```python
from build123d import *

# Parameters (mm, degrees)
SKETCH_1_W      = 160
SKETCH_1_H      = 100
EXTRUDE_4_DEPTH = 20
SKETCH_3_R      = 20
EXTRUDE_5_DEPTH = 35


with BuildPart() as part:
    # 草图1 → 凸台-拉伸4 (new body)
    with BuildSketch(Plane.XY):
        with Locations((-86.209434593, 50.003007896)):
            Rectangle(SKETCH_1_W, SKETCH_1_H)
    extrude(amount=-EXTRUDE_4_DEPTH)

    # 草图3 → 凸台-拉伸5 (add)
    with BuildSketch(Plane(origin=(0, 0, -20), x_dir=(-1, 0, 0), z_dir=(0, 0, -1))):
        with Locations(Location((46.209434593, 50.003007896, 0), (0, 0, 180))):
            Circle(SKETCH_3_R)
        with Locations(Location((126.209434593, 50.003007896, 0), (0, 0, 180))):
            Circle(SKETCH_3_R)
    extrude(amount=EXTRUDE_5_DEPTH)


solid = part.part
```
Source: CAD feature listing. Evaluate the final solid. Frame: model axes, mm. A direction names the side the tool comes from. Round coordinates to 2 decimals unless told otherwise and drop trailing zeros. Loops run counter-clockwise (first coordinate to the right, second up) from the corner with the lowest first, then second, coordinate; pieces in that order, holes last. Notation, with made-up numbers: M -34.75,80.5 L -25.75,80.5 A19 cw -25.75,111.5 Z; hole C -2,68 d4. An arc over 180 degrees is marked long. Use a Markdown table: item, result. Add a question column.
1. Cut plane D-D, the plane y = 32. Output: boundary loops of the cut face in (x, z).
2. Ray query, line 1 along Z through (x, y) = (-89.5, 66); line 2 along X through (y, z) = (52, -31); line 3 along X through (y, z) = (59, -25). Return the intervals inside material, ascending. Write a range as [from, to].
3. Cut plane B-B, the plane x = -120. Output: boundary loops of the cut face in (y, z).
4. Pull-direction query (X, two-part tool) for faces 3 (the flat face through (-87, 100.003, -10)), 4 (the flat face through (-166.209, 49, -10)), 5 (the cylindrical face through (-146.19, 49.12, -37.25)); classes: +X half, -X half, draft (parallel to the pull), parting line (faces both ways), or undercut.
5. Contact query for flat-ended pins moving along their axis: pin 1 (6 mm diameter, centred on x = -71.5, z = -35, fed in from -Y); pin 2 (2 mm diameter, centred on x = -62, z = -42.5, fed in from -Y); pin 3 (8 mm diameter, centred on y = 60.5, z = -25, fed in from -X); pin 4 (4 mm diameter, centred on x = -28, y = 35, fed in from -Z). Output: stop coordinate, or through.
6. Cut plane A-A, the plane y = 46. Output: boundary loops of the cut face in (x, z), and give its area (3 significant figures).
7. Set-up query: faces 1 (the flat face through (-87, 51, 0)), 2 (the flat face through (-87, 51, -20)). Return all of +Z, -Z, +X, -X, +Y, -Y with unobstructed straight access to the full face (end or side cutting, diameter ignored); none if empty.
8. Cut plane C-C, the plane z = -27. Output: boundary loops of the cut face in (x, y), and give its area (3 significant figures).
Solution:
| question | item | result |
|---|---|---|
| 1 | outline | M -166.21,-20 L -134.92,-20 L -134.92,-55 L -117.5,-55 L -117.5,-20 L -54.92,-20 L -54.92,-55 L -37.5,-55 L -37.5,-20 L -6.21,-20 L -6.21,0 L -166.21,0 Z |
| 2 | line 1 | z = [-20, 0] |
| 2 | line 2 | x = [-146.11, -106.31], [-66.11, -26.31] |
| 2 | line 3 | x = [-144.07, -108.35], [-64.07, -28.35] |
| 3 | outline | M 0,-20 L 30.99,-20 L 30.99,-55 L 69.01,-55 L 69.01,-20 L 100,-20 L 100,0 L 0,0 Z |
| 4 | face 3 | draft |
| 4 | face 4 | -X half |
| 4 | face 5 | undercut |
| 5 | pin 1 | passes through |
| 5 | pin 2 | stops at y = 36.54 |
| 5 | pin 3 | stops at x = -145.12 |
| 5 | pin 4 | stops at z = -20 |
| 6 | outline | M -166.21,-20 L -145.8,-20 L -145.8,-55 L -106.61,-55 L -106.61,-20 L -65.8,-20 L -65.8,-55 L -26.61,-55 L -26.61,-20 L -6.21,-20 L -6.21,0 L -166.21,0 Z |
| 6 | area | 5,940 mm2 |
| 7 | face 1 | +Z, +X, -X, +Y, -Y |
| 7 | face 2 | -Z |
| 8 | outline | C -126.21,50 d40; C -46.21,50 d40 |
| 8 | area | 2,510 mm2 |
